from build123d import *

# Parameters (mm, degrees)
SKETCH_1_R      = 2.25
EXTRUDE_1_DEPTH = 3


with BuildPart() as part:
    # 草图1 → 凸台-拉伸1 (new body)
    with BuildSketch(Plane(origin=(0, 0, 0), x_dir=(-1, 0, 0), z_dir=(0, 0, -1))):
        with BuildLine():
            Line((-46.697056051, -46.688916039), (-39.554488655, -47.948343383))
            ThreePointArc((-39.554488655, -47.948343383), (-39.277504317, -47.896375463), (-39.103531516, -47.674667428))
            ThreePointArc((-39.103531516, -47.674667428), (0, -19), (39.103531516, -47.674667428))
            ThreePointArc((39.103531516, -47.674667428), (39.277504317, -47.896375463), (39.554488655, -47.948343383))
            Line((39.554488655, -47.948343383), (46.697056051, -46.688916039))
            ThreePointArc((46.697056051, -46.688916039), (46.967515904, -46.505836455), (47.011363008, -46.182194526))
            ThreePointArc((47.011363008, -46.182194526), (41.589384656, -34.090096798), (33.125428162, -23.893130722))
            ThreePointArc((33.125428162, -23.893130722), (26.210916767, -14.399107105), (23.515754966, -2.967438148))
            ThreePointArc((23.515754966, -2.967438148), (23.211784398, -2.281473086), (22.516285244, -2))
            Line((22.516285244, -2), (16.5, -2))
            ThreePointArc((16.5, -2), (15.792893219, -2.292893219), (15.5, -3))
            Line((15.5, -3), (15.5, -9))
            ThreePointArc((15.5, -9), (15.207106781, -9.707106781), (14.5, -10))
            Line((14.5, -10), (-14.5, -10))
            ThreePointArc((-14.5, -10), (-15.207106781, -9.707106781), (-15.5, -9))
            Line((-15.5, -9), (-15.5, -3))
            ThreePointArc((-15.5, -3), (-15.792893219, -2.292893219), (-16.5, -2))
            Line((-16.5, -2), (-22.516285244, -2))
            ThreePointArc((-22.516285244, -2), (-23.211784398, -2.281473086), (-23.515754966, -2.967438148))
            ThreePointArc((-23.515754966, -2.967438148), (-26.210916767, -14.399107105), (-33.125428162, -23.893130722))
            ThreePointArc((-33.125428162, -23.893130722), (-41.589384656, -34.090096798), (-47.011363008, -46.182194526))
            ThreePointArc((-47.011363008, -46.182194526), (-46.967515904, -46.505836455), (-46.697056051, -46.688916039))
        make_face()
        with Locations(Location((-38.97114317, -37.5, 0), (0, 0, 180))):
            Circle(SKETCH_1_R, mode=Mode.SUBTRACT)
        with Locations(Location((19.5, -6, 0), (0, 0, 180))):
            Circle(SKETCH_1_R, mode=Mode.SUBTRACT)
        with Locations(Location((38.97114317, -37.5, 0), (0, 0, 180))):
            Circle(SKETCH_1_R, mode=Mode.SUBTRACT)
        with Locations(Location((0, -15, 0), (0, 0, 180))):
            Circle(SKETCH_1_R, mode=Mode.SUBTRACT)
        with Locations(Location((-19.5, -6, 0), (0, 0, 180))):
            Circle(SKETCH_1_R, mode=Mode.SUBTRACT)
    extrude(amount=-EXTRUDE_1_DEPTH)


solid = part.part
Geometry check sheet. Reference: the model listing, model coordinates, mm. A direction names the side the tool comes from. Round coordinates to 2 decimals unless told otherwise and drop trailing zeros. Write each loop counter-clockwise with the first axis right and the second up, starting at its lowest first coordinate (ties: lowest second). Pieces come first, ordered by that corner, then holes. Notation, with made-up numbers: (49, 24.25) -> (89, 24.25) arc R17 ccw to (89, 50.25) -> close; hole circle Ø1 at (-36.75, 28.5). An arc over 180 degrees is marked (long way). One line per item, written item: value. Start each with the question number.
(1) Cross-section at A-A, the plane z = 2. Record the cut outline in (x, y) (3 decimals), and give its area (3 significant figures).
(2) Draft check along Y on faces 3 (the flat face through (-20, -2, 1)), 4 (the cylindrical face through (0.726, -19.006, 1.479)), 5 (the cylindrical face through (40.18, -39.4, 1.48)). Enter one of: +Y half, -Y half, draft (parallel to the pull), parting line (faces both ways), or undercut.
(3) Access from +Z, -Z, +X, -X, +Y, -Y to the whole of each face (thin tool, end or side, straight path). Record for faces 1 (the flat face through (0, -10, 1)), 2 (the cylindrical face through (26.142, -14.248, 1.479)).
(4) Scan lines: line 1 (X direction, y = -37.5, z = 1); line 2 (X direction, y = -35.5, z = 2.55); line 3 (Y direction, x = 0, z = 1.3). Record each from-to range of solid material in increasing order. Write a range as [from, to].
(5) Go/stop test with flat-tipped pins: pin 1 Ø5 at (x, y) = (19.5, -6) entering from +Z; pin 2 Ø1 at (y, z) = (-21, 1.5) entering from +X; pin 3 Ø1.5 at (x, z) = (4.5, 1) entering from +Y; pin 4 Ø1.5 at (y, z) = (-5, 2) entering from -X. Record where each tip stops, or that it passes through.
(6) Cross-section at B-B, the plane x = 0. Record the cut outline in (y, z).
(7) Cross-section at C-C, the plane y = -34. Record the cut outline in (x, z).
(8) Cross-section at D-D, the plane y = -6. Record the cut outline in (x, z), and give its area (3 significant figures).
Answer:
1. outline: (-47.011, -46.182) arc R0.4 ccw to (-46.697, -46.689) -> (-39.554, -47.948) arc R0.4 ccw to (-39.104, -47.675) arc R41 cw to (39.104, -47.675) arc R0.4 ccw to (39.554, -47.948) -> (46.697, -46.689) arc R0.4 ccw to (47.011, -46.182) arc R49 ccw to (33.125, -23.893) arc R29.711 cw to (23.516, -2.967) arc R1 ccw to (22.516, -2) -> (16.5, -2) arc R1 ccw to (15.5, -3) -> (15.5, -9) arc R1 cw to (14.5, -10) -> (-14.5, -10) arc R1 cw to (-15.5, -9) -> (-15.5, -3) arc R1 ccw to (-16.5, -2) -> (-22.516, -2) arc R1 ccw to (-23.516, -2.967) arc R29.711 cw to (-33.125, -23.893) arc R49 ccw to start; hole circle Ø4.5 at (-38.971, -37.5); hole circle Ø4.5 at (-19.5, -6); hole circle Ø4.5 at (0, -15); hole circle Ø4.5 at (19.5, -6); hole circle Ø4.5 at (38.971, -37.5)
1. area: 1,170 mm²
2. face 3: +Y half
2. face 4: -Y half
2. face 5: undercut
3. face 1: +Z, -Z, +Y
3. face 2: +Z, -Z, +X, +Y
4. line 1: [-43.53, -41.22], [-36.72, -34.27], [34.27, 36.72], [41.22, 43.53]
4. line 2: [-42.44, -40], [-37.94, -32.87], [32.87, 37.94], [40, 42.44]
4. line 3: [-19, -17.25], [-12.75, -10]
5. pin 1: z = 3
5. pin 2: x = 30.79
5. pin 3: y = -10
5. pin 4: x = -23.74
6. outline: (-19, 0) -> (-17.25, 0) -> (-17.25, 3) -> (-19, 3) -> close; (-12.75, 0) -> (-10, 0) -> (-10, 3) -> (-12.75, 3) -> close
7. outline: (-41.53, 0) -> (-31.7, 0) -> (-31.7, 3) -> (-41.53, 3) -> close; (31.7, 0) -> (41.53, 0) -> (41.53, 3) -> (31.7, 3) -> close
8. outline: (-23.77, 0) -> (-21.75, 0) -> (-21.75, 3) -> (-23.77, 3) -> close; (-17.25, 0) -> (-15.5, 0) -> (-15.5, 3) -> (-17.25, 3) -> close; (15.5, 0) -> (17.25, 0) -> (17.25, 3) -> (15.5, 3) -> close; (21.75, 0) -> (23.77, 0) -> (23.77, 3) -> (21.75, 3) -> close
8. area: 22.6 mm²
